from build123d import *

# Parameters (mm, degrees)
F0_W     = 40
F0_H     = 40
F1_DEPTH = 20
F2_T     = -2.5
F3_R     = 4
F4_DEPTH = 40.001


with BuildPart() as f1:
    # F0 (on Right) → F1 (new body)
    with BuildSketch(Plane.YZ):
        with Locations((3.175765, 4.096127)):
            Rectangle(F0_W, F0_H)
    extrude(amount=F1_DEPTH)

    # F2
    f2_openings = [f1.faces().sort_by_distance(p)[0] for p in [
        (20, 3.175765, 4.096127),
    ]]
    offset(amount=F2_T, openings=f2_openings)

    # F3 (on face) → F4 (cut, through all)
    with BuildSketch(Plane(origin=(0, 0, -15.903873), x_dir=(1, 0, 0), z_dir=(0, 0, -1))):
        with Locations((14, -3.175765)):
            Circle(F3_R)
    extrude(amount=-F4_DEPTH, mode=Mode.SUBTRACT)


solid = f1.part
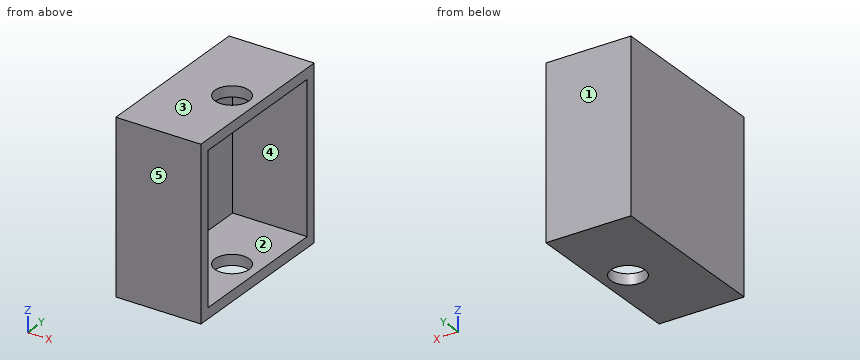
Verification items for the finished model (mm, model axes). Face numbers are marked on the shaded views. A direction names the side the tool comes from. Give positions to 0.01 mm unless a question says otherwise; leave off trailing zeros. Write each loop counter-clockwise with the first axis right and the second up, starting at its lowest first coordinate (ties: lowest second). Pieces come first, ordered by that corner, then holes.
(1) Gauge pin test, flat end, axial feed: pin 1 (10.5 mm diameter, centred on y = -1, z = 11, fed in from +X). Record the tip position at first contact, or that the pin passes through.
(2) Access from +Z, -Z, +X, -X, +Y, -Y to the whole of each face (thin tool, end or side, straight path). Record for the marked faces 4 and 5.
(3) Cross-section at A-A (x = 14). Enter the section's corners in (y, z), plus the area to 3 significant figures.
(4) Cross-section at B-B (y = 1). Enter the section's corners in (x, z).
(5) Cross-section at C-C (z = 2.5). Enter the section's corners in (x, y), plus the area to 4 significant figures.
(6) Cross-section at D-D (y = 9). Enter the section's corners in (x, z).
(7) Material ranges on line 1 (Y direction, x = 14, z = 22.2); line 2 (Y direction, x = 13, z = 17); line 3 (Z direction, x = 4.75, y = 17.5), recorded low to high.
(8) Mould release check, pull along Z, two halves, no side actions. Record for the marked faces 1, 2 and 3: +Z half, -Z half, draft (parallel to the pull), parting line (faces both ways), or undercut.
Worked out:
1. pin 1: stops at x = 2.5
2. face 4: +X
2. face 5: +Z, -Z, +X, -X, -Y
3. outline: (-16.82, -15.9) - (-0.82, -15.9) - (-0.82, -13.4) - (-14.32, -13.4) - (-14.32, 21.6) - (-0.82, 21.6) - (-0.82, 24.1) - (-16.82, 24.1) - close; (7.18, -15.9) - (23.18, -15.9) - (23.18, 24.1) - (7.18, 24.1) - (7.18, 21.6) - (20.68, 21.6) - (20.68, -13.4) - (7.18, -13.4) - close
3. area: 335 mm2
4. outline: (0, -15.9) - (10.64, -15.9) - (10.64, -13.4) - (2.5, -13.4) - (2.5, 21.6) - (10.64, 21.6) - (10.64, 24.1) - (0, 24.1) - close; (17.36, -15.9) - (20, -15.9) - (20, -13.4) - (17.36, -13.4) - close; (17.36, 21.6) - (20, 21.6) - (20, 24.1) - (17.36, 24.1) - close
5. outline: (0, -16.82) - (20, -16.82) - (20, -14.32) - (2.5, -14.32) - (2.5, 20.68) - (20, 20.68) - (20, 23.18) - (0, 23.18) - close
5. area: 187.5 mm2
6. outline: (0, -15.9) - (20, -15.9) - (20, -13.4) - (2.5, -13.4) - (2.5, 21.6) - (20, 21.6) - (20, 24.1) - (0, 24.1) - close
7. line 1: y = -16.82 to -0.82, 7.18 to 23.18
7. line 2: y = -16.82 to -14.32, 20.68 to 23.18
7. line 3: z = -15.9 to -13.4, 21.6 to 24.1
8. face 1: draft
8. face 2: undercut
8. face 3: +Z half
